from build123d import *

# Parameters (mm, degrees)
ESQUISSE1_R        = 8
ESQUISSE1_R_2      = 5
BOSS_EXTRU_2_DEPTH = 10


with BuildPart() as part:
    # Esquisse1 → Boss.-Extru.2 (new body)
    with BuildSketch(Plane(origin=(0, 0, 0), x_dir=(1, 0, 0), z_dir=(0, 1, 0))):
        with BuildLine():
            Line((88.589203043, -110.181902046), (139.966204056, -19.938910608))
            ThreePointArc((139.966204056, -19.938910608), (144.170152865, -15.949329734), (149.881071002, -14.961729023))
            ThreePointArc((149.881071002, -14.961729023), (167.84005434, 1.014572883), (149.689240839, 16.772595422))
            ThreePointArc((149.689240839, 16.772595422), (143.966800629, 17.691082861), (139.71492773, 21.629549313))
            Line((139.71492773, 21.629549313), (87.250705139, 111.24483308))
            ThreePointArc((87.250705139, 111.24483308), (85.897601156, 116.880349981), (87.897772919, 122.319950523))
            ThreePointArc((87.897772919, 122.319950523), (83.04138128, 145.861037272), (60.319126696, 138.02098295))
            ThreePointArc((60.319126696, 138.02098295), (56.662473136, 133.524448077), (51.125724688, 131.811451359))
            Line((51.125724688, 131.811451359), (-52.715498918, 131.183743688))
            ThreePointArc((-52.715498918, 131.183743688), (-58.272551709, 132.829679716), (-61.983298082, 137.281679546))
            ThreePointArc((-61.983298082, 137.281679546), (-84.79867306, 144.846464389), (-89.370114142, 121.248387528))
            ThreePointArc((-89.370114142, 121.248387528), (-87.304327493, 115.833365215), (-88.589203043, 110.181902046))
            Line((-88.589203043, 110.181902046), (-139.966204056, 19.938910608))
            ThreePointArc((-139.966204056, 19.938910608), (-144.170152865, 15.949329734), (-149.881071002, 14.961729023))
            ThreePointArc((-149.881071002, 14.961729023), (-167.84005434, -1.014572883), (-149.689240839, -16.772595422))
            ThreePointArc((-149.689240839, -16.772595422), (-143.966800629, -17.691082861), (-139.71492773, -21.629549313))
            Line((-139.71492773, -21.629549313), (-87.250705139, -111.24483308))
            ThreePointArc((-87.250705139, -111.24483308), (-85.897601156, -116.880349981), (-87.897772919, -122.319950523))
            ThreePointArc((-87.897772919, -122.319950523), (-83.04138128, -145.861037272), (-60.319126696, -138.02098295))
            ThreePointArc((-60.319126696, -138.02098295), (-56.662473136, -133.524448077), (-51.125724688, -131.811451359))
            Line((-51.125724688, -131.811451359), (52.715498918, -131.183743688))
            ThreePointArc((52.715498918, -131.183743688), (58.272551709, -132.829679716), (61.983298082, -137.281679546))
            ThreePointArc((61.983298082, -137.281679546), (84.79867306, -144.846464389), (89.370114142, -121.248387528))
            ThreePointArc((89.370114142, -121.248387528), (87.304327493, -115.833365215), (88.589203043, -110.181902046))
        make_face()
        with Locations(Location((-151.840346656, -0.91785658, 0), (0, 0, 270))):  # turned: the seam where the file's is
            Circle(ESQUISSE1_R, mode=Mode.SUBTRACT)
        with Locations(Location((-76.715060443, 131.038669234, 0), (0, 0, 270))):  # turned: the seam where the file's is
            Circle(ESQUISSE1_R, mode=Mode.SUBTRACT)
        with Locations(Location((75.125286213, 131.956525813, 0), (0, 0, 270))):  # turned: the seam where the file's is
            Circle(ESQUISSE1_R, mode=Mode.SUBTRACT)
        with Locations(Location((151.840346656, 0.91785658, 0), (0, 0, 270))):  # turned: the seam where the file's is
            Circle(ESQUISSE1_R, mode=Mode.SUBTRACT)
        with Locations(Location((76.715060443, -131.038669234, 0), (0, 0, 270))):  # turned: the seam where the file's is
            Circle(ESQUISSE1_R, mode=Mode.SUBTRACT)
        with Locations(Location((-75.125286213, -131.956525813, 0), (0, 0, 270))):  # turned: the seam where the file's is
            Circle(ESQUISSE1_R, mode=Mode.SUBTRACT)
        with Locations(Location((0, 70, 0), (0, 0, 270))):  # turned: the seam where the file's is
            Circle(ESQUISSE1_R, mode=Mode.SUBTRACT)
        with Locations(Location((60.621778265, -35, 0), (0, 0, 270))):  # turned: the seam where the file's is
            Circle(ESQUISSE1_R, mode=Mode.SUBTRACT)
        with Locations(Location((-60.621778265, -35, 0), (0, 0, 270))):  # turned: the seam where the file's is
            Circle(ESQUISSE1_R, mode=Mode.SUBTRACT)
        with Locations(Location((0, 0, 0), (0, 0, 270))):  # turned: the seam where the file's is
            Circle(ESQUISSE1_R_2, mode=Mode.SUBTRACT)
    extrude(amount=-BOSS_EXTRU_2_DEPTH)


solid = part.part
Design review of the part built by this model. Coordinates are the model's own, in mm. A direction names the side the tool comes from. Give positions to 0.01 mm unless a question says otherwise; leave off trailing zeros. Loops run counter-clockwise (first coordinate to the right, second up) from the corner with the lowest first, then second, coordinate; pieces in that order, holes last. Notation, with made-up numbers: (44.5, 17) - (73.5, 17) arc R29 ccw to (73.5, 42) - close; hole circle Ø11 at (53, 78.25). An arc over 180 degrees is marked (long way). Write item = value, one per line.
1) Take a section at A-A on x = 56.5. State the section outline as (y, z) points, and give its area (3 significant figures).
Result sheet:
outline = (-10, -133.42) - (0, -133.42) - (0, 28.14) - (-10, 28.14) - close; (-10, 41.86) - (0, 41.86) - (0, 131.9) - (-10, 131.9) - close
area = 2,520 mm2
2) To check wall thickness, follow line 1 (Z direction, x = -151, y = -0.75); line 2 (Z direction, x = -68, y = -3.5); line 3 (X direction, y = -2.25, z = -126.5). State the ranges of each line that lie inside material, in increasing order.
Result sheet:
line_1 = -15.06 to -7.04, 8.87 to 16.9
line_2 = -144.46 to 31.91, 38.09 to 128.32, 135.59 to 146.28
line_3 = -92.06 to -83.3, -70.13 to 69.27, 80.98 to 90.17
3) Clearance check with flat-ended pins moving along their axes: pin 1 Ø8 at (x, z) = (0, 0) entering from +Y; pin 2 Ø1.5 at (y, z) = (-4.5, -43.5) entering from +X; pin 3 Ø3 at (x, y) = (105.5, -5.5) entering from +Z; pin 4 Ø1 at (x, y) = (-38, -4.5) entering from +Z. State where each tip first meets the part, or that it passes through.
Result sheet:
pin_1 = through
pin_2 = 127.35
pin_3 = 83.11
pin_4 = 131.74
4) Take a section at C-C on z = 36.5. State the section outline as (x, y) points, and give its area (3 significant figures).
Result sheet:
outline = (-131.01, -10) - (-68.48, -10) - (-68.48, 0) - (-131.01, 0) - close; (-52.76, -10) - (52.76, -10) - (52.76, 0) - (-52.76, 0) - close; (68.48, -10) - (130.54, -10) - (130.54, 0) - (68.48, 0) - close
area = 2,300 mm2
5) Draft analysis for pull direction Z (two halves, no side actions). For faces 4 (the face through (66.029, -4.93, 29.104)), 5 (the face through (56.73, -4.93, -133.57)), 6 (the face through (-56.73, -4.93, 133.57)), 7 (the face through (167.838, -4.93, -0.634)), state which applies: +Z half, -Z half, draft (parallel to the pull), parting line (faces both ways), or undercut.
Result sheet:
face_4 = undercut
face_5 = -Z half
face_6 = +Z half
face_7 = parting line
6) Tool access review of faces 1 (the face through (-58.204, -4.93, -132.785)), 2 (the face through (58.204, -4.93, 132.785)), 3 (the face through (-4.868, -4.93, -76.349)): name each direction out of +Z, -Z, +X, -X, +Y, -Y from which nothing blocks a thin tool from reaching the whole face with its end or side.
Result sheet:
face_1 = -Z, +Y, -Y
face_2 = +Z, +Y, -Y
face_3 = +Y, -Y
7) Take a section at D-D on y = -3. Count the separate pieces of the cut face and the enclosed holes in it, and give its area (3 significant figures).
Result sheet:
separate_pieces = 1
enclosed_holes = 10
area = 61,400 mm2
8) Take a section at B-B on z = 0. State the section outline as (x, y) points.
Result sheet:
outline = (-167.81, -10) - (-159.79, -10) - (-159.79, 0) - (-167.81, 0) - close; (-143.89, -10) - (-5, -10) - (-5, 0) - (-143.89, 0) - close; (5, -10) - (143.89, -10) - (143.89, 0) - (5, 0) - close; (159.79, -10) - (167.81, -10) - (167.81, 0) - (159.79, 0) - close
